Design review of the part built by this model. Coordinates are the model's own, in mm. Face numbers are marked on the shaded views. A direction names the side the tool comes from. Give positions to 0.01 mm unless a question says otherwise; leave off trailing zeros. Write each loop counter-clockwise with the first axis right and the second up, starting at its lowest first coordinate (ties: lowest second). Pieces come first, ordered by that corner, then holes.
```python
from build123d import *

# Parameters (mm, degrees)
BOSS_EXTRUDE1_DEPTH = 11.6
CUT_EXTRUDE1_DEPTH  = 9.55
SKETCH5_W           = 27
SKETCH5_H           = 11.6
CUT_EXTRUDE3_DEPTH  = 51.592094244
CUT_EXTRUDE4_DEPTH  = 3
CUT_EXTRUDE5_DEPTH  = 9.55
SKETCH8_R           = 1.26
CUT_EXTRUDE6_DEPTH  = 4
SKETCH9_W           = 29
SKETCH9_H           = 7.5
CUT_EXTRUDE7_DEPTH  = 51.592094244
SKETCH10_R          = 0.75
CUT_EXTRUDE8_DEPTH  = 4
SKETCH11_R          = 1
CUT_EXTRUDE9_DEPTH  = 4


with BuildPart() as part:
    # Sketch2 → Boss-Extrude1 (new body)
    with BuildSketch(Plane(origin=(0, 0, 0), x_dir=(1, 0, 0), z_dir=(0, 1, 0))):
        Polygon((0, 5.767018283), (0, -6.232981717), (11, -20), (45, -20), (45, 20), (11, 20), align=None)
    extrude(amount=BOSS_EXTRUDE1_DEPTH)

    # Sketch3 → Cut-Extrude1 (cut)
    with BuildSketch(Plane(origin=(0, 11.6, 0), x_dir=(1, 0, 0), z_dir=(0, 1, 0))):
        Polygon((1.5, 7.707879426), (1.5, -8.110302392), (9.5, -18.122679325), (9.5, 18.059138857), align=None)
    extrude(amount=-CUT_EXTRUDE1_DEPTH, mode=Mode.SUBTRACT)

    # Sketch5 → Cut-Extrude3 (cut, through all)
    with BuildSketch(Plane(origin=(0, 11.6, 0), x_dir=(1, 0, 0), z_dir=(0, 1, 0))):
        with Locations((24, 0)):
            Rectangle(SKETCH5_W, SKETCH5_H)
    extrude(amount=-CUT_EXTRUDE3_DEPTH, mode=Mode.SUBTRACT)

    # Sketch6 → Cut-Extrude4 (cut)
    with BuildSketch(Plane(origin=(10.5, 0, 0), x_dir=(0, 0, -1), z_dir=(1, 0, 0))):
        with BuildLine():
            Line((2.5, 6.75), (2.5, 11.6))
            Line((2.5, 11.6), (-2.5, 11.6))
            Line((-2.5, 11.6), (-2.5, 6.75))
            ThreePointArc((-2.5, 6.75), (0, 4.25), (2.5, 6.75))
        make_face()
    extrude(amount=-CUT_EXTRUDE4_DEPTH, mode=Mode.SUBTRACT)

    # Sketch7 → Cut-Extrude5 (cut)
    with BuildSketch(Plane(origin=(0, 11.6, 0), x_dir=(1, 0, 0), z_dir=(0, 1, 0))):
        Polygon((1.5, 7.707879426), (0, 5.767018283), (1.5, 5.767018283), align=None)
        Polygon((0, -6.232981717), (1.5, -6.232981717), (1.5, -8.110302392), align=None)
    extrude(amount=-CUT_EXTRUDE5_DEPTH, mode=Mode.SUBTRACT)

    # Sketch8 → Cut-Extrude6 (cut)
    with BuildSketch(Plane.XZ):
        with Locations(Location((30.5, 9.89, 0), (0, 0, 270))):
            Circle(SKETCH8_R)
        with Locations(Location((30.5, -9.89, 0), (0, 0, 270))):
            Circle(SKETCH8_R)
    extrude(amount=-CUT_EXTRUDE6_DEPTH, mode=Mode.SUBTRACT)

    # Sketch9 → Cut-Extrude7 (cut, through all)
    with BuildSketch(Plane.XZ):
        with Locations((30.5, 16.25)):
            Rectangle(SKETCH9_W, SKETCH9_H)
        with Locations((30.5, -16.25)):
            Rectangle(SKETCH9_W, SKETCH9_H)
    extrude(amount=-CUT_EXTRUDE7_DEPTH, mode=Mode.SUBTRACT)

    # Sketch10 → Cut-Extrude8 (cut)
    with BuildSketch(Plane(origin=(0, 11.6, 0), x_dir=(1, 0, 0), z_dir=(0, 1, 0))):
        with Locations(Location((13.5, 16.5, 0), (0, 0, 270))):
            Circle(SKETCH10_R)
        with Locations(Location((13.5, 9, 0), (0, 0, 270))):
            Circle(SKETCH10_R)
        with Locations(Location((41.5, 9, 0), (0, 0, 270))):
            Circle(SKETCH10_R)
        with Locations(Location((41.5, -9.3, 0), (0, 0, 270))):
            Circle(SKETCH10_R)
        with Locations(Location((13.5, -9.3, 0), (0, 0, 270))):
            Circle(SKETCH10_R)
        with Locations(Location((13.5, -16.5, 0), (0, 0, 270))):
            Circle(SKETCH10_R)
    extrude(amount=-CUT_EXTRUDE8_DEPTH, mode=Mode.SUBTRACT)

    # Sketch11 → Cut-Extrude9 (cut)
    with BuildSketch(Plane(origin=(45, 0, 0), x_dir=(0, 0, -1), z_dir=(1, 0, 0))):
        with Locations((-8.5, 6)):
            Circle(SKETCH11_R)
        with Locations((1.5, 6)):
            Circle(SKETCH11_R)
    extrude(amount=-CUT_EXTRUDE9_DEPTH, mode=Mode.SUBTRACT)


solid = part.part
```
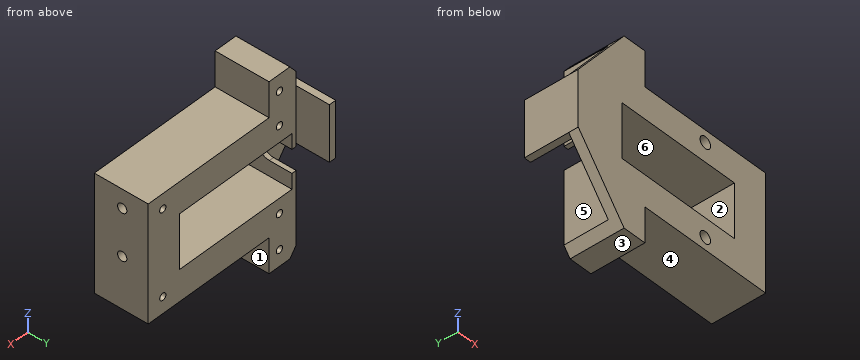
(1) Mouldability with a two-part tool opening along X and no side actions: class the marked faces 1, 2 and 3 as pulls with the +X half, pulls with the -X half, needs draft (parallel to the pull), parting line crosses it, or undercut.
Resolved:
face 1: pulls with the +X half
face 2: undercut
face 3: needs draft
(2) Clearance check with flat-ended pins moving along their axes: P1, Ø0.8, axis at x = 10, y = 10.5, coming from the -Z side; P2, Ø1.5, axis at x = 27, y = 10, coming from the +Z side; P3, Ø1, axis at y = 6, z = -1.5, coming from the +X side; P4, Ø1, axis at x = 24, z = 3.5, coming from the +Y side. State where each tip first meets the part, or that it passes through.
Resolved:
P1: stops at z = -19.22
P2: stops at z = 12.5
P3: stops at x = 41
P4: passes through
(3) Consider section B-B, the plane x = 13.5. Give the boundary of the cut face in (y, z).
Resolved:
outline: (0, -20) - (11.6, -20) - (11.6, -17.25) - (7.6, -17.25) - (7.6, -15.75) - (11.6, -15.75) - (11.6, -9.75) - (7.6, -9.75) - (7.6, -8.25) - (11.6, -8.25) - (11.6, -5.8) - (0, -5.8) - close; (0, 5.8) - (11.6, 5.8) - (11.6, 8.55) - (7.6, 8.55) - (7.6, 10.05) - (11.6, 10.05) - (11.6, 15.75) - (7.6, 15.75) - (7.6, 17.25) - (11.6, 17.25) - (11.6, 20) - (0, 20) - close
(4) Consider section A-A, the plane z = 0. Give the boundary of the cut face in (x, y), then the cut area to 3 significant figures.
Resolved:
outline: (0, 0) - (10.5, 0) - (10.5, 4.25) - (9.5, 4.25) - (9.5, 2.05) - (1.5, 2.05) - (1.5, 11.6) - (0, 11.6) - close; (37.5, 0) - (45, 0) - (45, 11.6) - (37.5, 11.6) - close
area: 125 mm2
(5) To check wall thickness, follow L1, parallel to X at y = 10, z = 9.3; L2, parallel to X at y = 9.75, z = -16.5; L3, parallel to Z at x = 34, y = 11.25. State the ranges of each line that lie inside material, in increasing order.
Resolved:
L1: x = 9.5 to 12.75, 14.25 to 40.75, 42.25 to 45
L2: x = 9.5 to 12.75, 14.25 to 16
L3: z = -12.5 to -5.8, 5.8 to 12.5
(6) Tool access review of the marked faces 4, 5 and 6: name each direction out of +Z, -Z, +X, -X, +Y, -Y from which nothing blocks a thin tool from reaching the whole face with its end or side.
Resolved:
face 4: -Z, +X, +Y, -Y
face 5: +Z, -Z, +Y
face 6: +Y, -Y
(7) Consider section D-D, the plane x = 41.5. Give the boundary of the cut face in (y, z).
Resolved:
outline: (0, -12.5) - (11.6, -12.5) - (11.6, -9.75) - (7.6, -9.75) - (7.6, -8.25) - (11.6, -8.25) - (11.6, 8.55) - (7.6, 8.55) - (7.6, 10.05) - (11.6, 10.05) - (11.6, 12.5) - (0, 12.5) - close; hole circle Ø2 at (6, -1.5); hole circle Ø2 at (6, 8.5)
